from build123d import *

# Parameters (mm, degrees)
BOSS_EXTRUDE1_START = 2.5
SKETCH1_R           = 1.6
BOSS_EXTRUDE1_DEPTH = 2


with BuildPart() as part:
    # Sketch1 → Boss-Extrude1 (new body)
    with BuildSketch(Plane.XY.offset(BOSS_EXTRUDE1_START)):
        with BuildLine():
            Line((-36.508029185, -42.375), (-36.508029185, -94.025))
            ThreePointArc((-36.508029185, -94.025), (-36.303003932, -94.519974747), (-35.808029185, -94.725))
            Line((-35.808029185, -94.725), (28.491970815, -94.725))
            ThreePointArc((28.491970815, -94.725), (28.986945562, -94.519974747), (29.191970815, -94.025))
            Line((29.191970815, -94.025), (29.191970815, -92.714949494))
            ThreePointArc((29.191970815, -92.714949494), (29.245255142, -92.447071091), (29.396996068, -92.219974747))
            Line((29.396996068, -92.219974747), (31.691970815, -89.925))
            Line((31.691970815, -89.925), (31.691970815, -57.025))
            Line((31.691970815, -57.025), (29.396996068, -54.730025253))
            ThreePointArc((29.396996068, -54.730025253), (29.245255142, -54.502928909), (29.191970815, -54.235050506))
            Line((29.191970815, -54.235050506), (29.191970815, -41.675))
            Line((29.191970815, -41.675), (-35.808029185, -41.675))
            ThreePointArc((-35.808029185, -41.675), (-36.303003932, -41.880025253), (-36.508029185, -42.375))
        make_face()
        with Locations((-21.508029185, -44.025)):
            Circle(SKETCH1_R, mode=Mode.SUBTRACT)
        with Locations((-22.908029185, -92.325)):
            Circle(SKETCH1_R, mode=Mode.SUBTRACT)
        with Locations((29.291970815, -59.175)):
            Circle(SKETCH1_R, mode=Mode.SUBTRACT)
        with Locations((29.291970815, -87.125)):
            Circle(SKETCH1_R, mode=Mode.SUBTRACT)
    extrude(amount=BOSS_EXTRUDE1_DEPTH)


solid = part.part
CAD build for the part. Positions are in the model's coordinates, mm. A direction names the side the tool comes from. Round coordinates to 2 decimals unless told otherwise and drop trailing zeros. Write each loop counter-clockwise with the first axis right and the second up, starting at its lowest first coordinate (ties: lowest second). Pieces come first, ordered by that corner, then holes.
(1) Slice it at A-A, the plane z = 3.3. Write the cut outline in (x, y) (3 decimals), and give its area (3 significant figures).
(2) Drop a flat-ended pin along its axis: P1, Ø2.5, axis at x = 29.29, y = -87.12, coming from the +Z side. Give the stop position or say it passes through.
(3) 3-axis set-ups, long thin cutter, end or side, ignore diameter. For faces 1 (the face through (29.192, -48, 3)), 2 (the face through (-4, -94.725, 3)), 3 (the face through (29.192, -93, 3)): which of +Z, -Z, +X, -X, +Y, -Y reach the whole face in a straight line?
(4) Slice it at B-B, the plane y = -52.5. Write the cut outline in (x, z), and give its area (3 significant figures).
(5) Probe line 1 along Y through (x, z) = (-22.5, 3.05) (3 decimals); line 2 along X through (y, z) = (-46, 4.05); line 3 along X through (y, z) = (-44.5, 3.3). List the from-to ranges inside material, lowest first.
(6) Mould opens along X. For faces 4 (the face through (31.692, -74, 3)), 5 (the face through (-3, -68, 4.5)), 6 (the face through (-36.508, -68, 3)), 7 (the face through (-23.12, -90.74, 3.49)) say: pulls with the +X half, pulls with the -X half, needs draft (parallel to the pull), parting line crosses it, or undercut.
From the geometry:
1. outline: (-36.508, -94.025) arc R0.7 ccw to (-35.808, -94.725) - (28.492, -94.725) arc R0.7 ccw to (29.192, -94.025) - (29.192, -92.715) arc R0.7 cw to (29.397, -92.22) - (31.692, -89.925) - (31.692, -57.025) - (29.397, -54.73) arc R0.7 cw to (29.192, -54.235) - (29.192, -41.675) - (-35.808, -41.675) arc R0.7 ccw to (-36.508, -42.375) - close; hole circle Ø3.2 at (-22.908, -92.325); hole circle Ø3.2 at (-21.508, -44.025); hole circle Ø3.2 at (29.292, -87.125); hole circle Ø3.2 at (29.292, -59.175)
1. area: 3,540 mm2
2. P1: passes through
3. face 1: +Z, -Z, +X, +Y
3. face 2: +Z, -Z, +X, -X, -Y
3. face 3: +Z, -Z, +X, -Y
4. outline: (-36.51, 2.5) - (29.19, 2.5) - (29.19, 4.5) - (-36.51, 4.5) - close
4. area: 131 mm2
5. line 1: y = -94.725 to -93.872, -90.778 to -45.28, -42.77 to -41.675
5. line 2: x = -36.51 to 29.19
5. line 3: x = -36.51 to -23.04, -19.98 to 29.19
6. face 4: pulls with the +X half
6. face 5: needs draft
6. face 6: pulls with the -X half
6. face 7: undercut
